from build123d import *

# Parameters (mm, degrees)
F0_R     = 12.95
F1_DEPTH = 3


with BuildPart() as f1:
    # F0 (on Top) → F1 (new body)
    with BuildSketch(Plane.XY):
        with BuildLine():
            ThreePointArc((34.99464, 0), (41.136207, 23.75), (17.49732, 30.306247))
            ThreePointArc((17.49732, 30.306247), (0, 47.5), (-17.49732, 30.306247))
            ThreePointArc((-17.49732, 30.306247), (-41.136207, 23.75), (-34.99464, 0))
            ThreePointArc((-34.99464, 0), (-41.136207, -23.75), (-17.49732, -30.306247))
            ThreePointArc((-17.49732, -30.306247), (0, -47.5), (17.49732, -30.306247))
            ThreePointArc((17.49732, -30.306247), (41.136207, -23.75), (34.99464, 0))
        make_face()
        with Locations((-25.980762, -15)):
            Circle(F0_R, mode=Mode.SUBTRACT)
        with Locations((0, -30)):
            Circle(F0_R, mode=Mode.SUBTRACT)
        with Locations((25.980762, -15)):
            Circle(F0_R, mode=Mode.SUBTRACT)
        with Locations((-25.980762, 15)):
            Circle(F0_R, mode=Mode.SUBTRACT)
        with BuildLine():
            ThreePointArc((-5.5, 9.526279), (0, 11), (5.5, 9.526279))
            ThreePointArc((5.5, 9.526279), (9.526279, 5.5), (11, 0))
            ThreePointArc((11, 0), (9.526279, -5.5), (5.5, -9.526279))
            ThreePointArc((5.5, -9.526279), (0, -11), (-5.5, -9.526279))
            ThreePointArc((-5.5, -9.526279), (-9.526279, -5.5), (-11, 0))
            ThreePointArc((-11, 0), (-9.526279, 5.5), (-5.5, 9.526279))
        make_face(mode=Mode.SUBTRACT)
        with Locations((25.980762, 15)):
            Circle(F0_R, mode=Mode.SUBTRACT)
        with Locations((0, 30)):
            Circle(F0_R, mode=Mode.SUBTRACT)
    extrude(amount=F1_DEPTH)


solid = f1.part
The listing builds one solid part. Answer for the finished solid, in the listing's coordinates (mm). Give positions to 0.01 mm unless a question says otherwise; leave off trailing zeros. Write each loop counter-clockwise with the first axis right and the second up, starting at its lowest first coordinate (ties: lowest second). Pieces come first, ordered by that corner, then holes. Notation, with made-up numbers: (10, 10) - (53, 10) arc R27 ccw to (53, 48) - close; hole circle Ø3 at (-16.5, 27). An arc over 180 degrees is marked (long way). Use a Markdown table: item, result.
1. Find the intervals of material crossed by probe 1 along Y at (x, z) = (15, 2.8); probe 2 along Y at (x, z) = (-0.5, 0.6); probe 3 along Y at (x, z) = (31, 0.75), in increasing order. Write a range as from..to.
Values follow:
| item | result |
|---|---|
| probe 1 | y = -39.01..-21.86, -8.14..8.14, 21.86..39.01 |
| probe 2 | y = -47.49..-42.94, -17.06..-10.99, 10.99..17.06, 42.94..47.49 |
| probe 3 | y = -31.76..-26.94, -3.06..3.06, 26.94..31.76 |
2. Section B-B on y = 15 is taken. Write down the section's boundary in (x, z).
Values follow:
| item | result |
|---|---|
| outline | (-43.48, 0) - (-38.93, 0) - (-38.93, 3) - (-43.48, 3) - close; (-13.03, 0) - (13.03, 0) - (13.03, 3) - (-13.03, 3) - close; (38.93, 0) - (43.48, 0) - (43.48, 3) - (38.93, 3) - close |
3. Section D-D on y = -24.5 is taken. Write down the section's boundary in (x, z).
Values follow:
| item | result |
|---|---|
| outline | (-40.68, 0) - (-34.78, 0) - (-34.78, 3) - (-40.68, 3) - close; (-17.18, 0) - (-11.72, 0) - (-11.72, 3) - (-17.18, 3) - close; (11.72, 0) - (17.18, 0) - (17.18, 3) - (11.72, 3) - close; (34.78, 0) - (40.68, 0) - (40.68, 3) - (34.78, 3) - close |
4. Section A-A on x = 0 is taken. Write down the section's boundary in (y, z), plus the area to 3 significant figures.
Values follow:
| item | result |
|---|---|
| outline | (-47.5, 0) - (-42.95, 0) - (-42.95, 3) - (-47.5, 3) - close; (-17.05, 0) - (-11, 0) - (-11, 3) - (-17.05, 3) - close; (11, 0) - (17.05, 0) - (17.05, 3) - (11, 3) - close; (42.95, 0) - (47.5, 0) - (47.5, 3) - (42.95, 3) - close |
| area | 63.6 mm² |
5. For a pull along X with two mould halves and no side action, classify faces 1 (the flat face through (-10, -7, 3)), 2 (the cylindrical face through (12.35, 33.89, 1.48)), 3 (the cylindrical face through (40.94, -24.08, 1.48)) as released by +X, released by -X, zero draft, split by the parting line, or undercut.
Values follow:
| item | result |
|---|---|
| face 1 | zero draft |
| face 2 | undercut |
| face 3 | undercut |
